Verification items for the finished model (mm, model axes). Coordinates: 2 decimals unless noted, no trailing zeros. Loops run counter-clockwise (first coordinate to the right, second up) from the corner with the lowest first, then second, coordinate; pieces in that order, holes last. Notation, with made-up numbers: (-32.75, -18) -> (-0.75, -18) arc R24 cw to (-0.75, 16) -> close; hole circle Ø8 at (53, 27.25). An arc over 180 degrees is marked (long way). Write item = value, one per line.
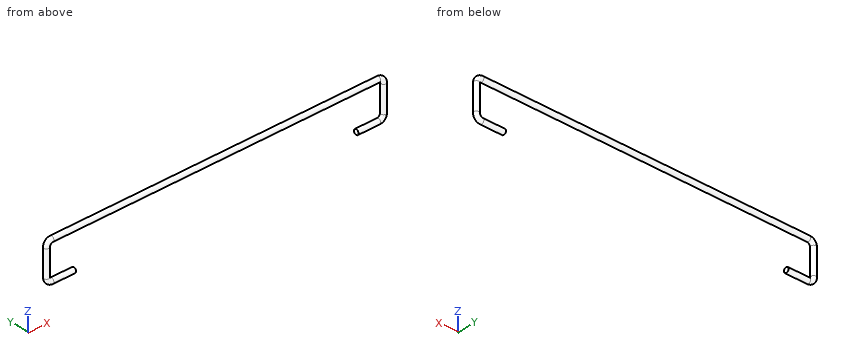
```python
from build123d import *

# Parameters (mm, degrees)
SEGMENT_R = 0.8


with BuildPart() as part:
    # Wire 2: sweep along a path in Path
    with BuildLine(Plane(origin=(0, 0, 0), x_dir=(1, 0, 0), z_dir=(0, 1, 0))) as wire_2_path:
        Line((-43.75, 11.5), (-50.6, 11.5))
        ThreePointArc((-50.6, 11.5), (-51.73137085, 11.03137085), (-52.2, 9.9))
        Line((-52.2, 9.9), (-52.2, 1.6))
        ThreePointArc((-52.2, 1.6), (-51.73137085, 0.46862915), (-50.6, 0))
        Line((-50.6, 0), (50.6, 0))
        ThreePointArc((50.6, 0), (51.73137085, 0.46862915), (52.2, 1.6))
        Line((52.2, 1.6), (52.2, 9.9))
        ThreePointArc((52.2, 9.9), (51.73137085, 11.03137085), (50.6, 11.5))
        Line((50.6, 11.5), (43.75, 11.5))
    # Segment → Wire 2 (sweep)
    with BuildSketch(Plane(origin=(-43.75, 0, 0), x_dir=(0, 0, -1), z_dir=(1, 0, 0))):
        with Locations((11.5, 0)):
            Circle(SEGMENT_R)
    sweep(path=wire_2_path.line)


solid = part.part
```
1) Depth check by flat-ended pin: pin 1 Ø0.8 at (y, z) = (-0.5, -11.5) entering from -X; pin 2 Ø0.8 at (y, z) = (0, -11.5) entering from +X. Enter the tip coordinate at first touch or a pass-through.
Ans:
pin_1 = -52.58
pin_2 = 52.68
2) Sectioned sample at B-B, the plane z = -6. Record the cut outline in (x, y).
Ans:
outline = circle Ø1.6 at (-52.2, 0); circle Ø1.6 at (52.2, 0)
3) Sectioned sample at C-C, the plane x = 1. Record the cut outline in (y, z).
Ans:
outline = circle Ø1.6 at (0, 0)
4) Sectioned sample at A-A, the plane x = 47.5. Record the cut outline in (y, z), plus the area to 3 significant figures.
Ans:
outline = circle Ø1.6 at (0, -11.5); circle Ø1.6 at (0, 0)
area = 4.02 mm2
5) Material ranges on line 1 (Z direction, x = -1, y = 0.1); line 2 (X direction, y = 0.5, z = -8.25); line 3 (X direction, y = -0.2, z = -1.5), recorded low to high.
Ans:
line_1 = -0.79 to 0.79
line_2 = -52.82 to -51.58, 51.58 to 52.82
line_3 = -52.97 to -51.42, 51.42 to 52.97
